Source: CAD feature listing. Evaluate the final solid. Frame: model axes, mm. Round coordinates to 2 decimals unless told otherwise and drop trailing zeros. Write each loop counter-clockwise with the first axis right and the second up, starting at its lowest first coordinate (ties: lowest second). Pieces come first, ordered by that corner, then holes. Notation, with made-up numbers: M 5,54 L 11,54 A18 ccw 11,83 Z; hole C 65,87.5 d2. An arc over 180 degrees is marked long. Answer in a Markdown table with one row per item. Add a question column.
Item 1: Cut plane B-B on z = 32. Return loops of the section in (x, y), and give its area (3 significant figures).
Item 2: Cut plane C-C on x = -46. Return loops of the section in (y, z), and give its area (3 significant figures).
Item 3: Material intervals for probe 1 along Z at (x, y) = (-29.5, -34); probe 2 along Z at (x, y) = (-50.5, -35.5); probe 3 along X at (y, z) = (-30, 29), sorted ascending.
Item 4: Contact query for flat-ended pins moving along their axis: pin 1 (4 mm diameter, centred on y = -12.5, z = 26.5, fed in from +X); pin 2 (3 mm diameter, centred on y = -20.5, z = 32, fed in from +X); pin 3 (10 mm diameter, centred on x = -28.5, y = -29, fed in from +Z). Output: stop coordinate, or through.
Item 5: Cut plane A-A on y = -12. Return loops of the section in (x, z), and give its area (3 significant figures).
from build123d import *

# Parameters (mm, degrees)
F0_W     = 25.4
F0_H     = 63.5
F1_DEPTH = 38.1


# Not quite as in the source:
# - a feature names something its author has since deleted; it is built from what else it names


with BuildPart() as f1:
    # F0 (on Front) → F1 (new body)
    with BuildSketch(Plane.XZ):
        Polygon((-101.6, 63.5), (-101.6, 0), (-29.9632605165, 0), (0, 0), (0, 12.7), align=None)
        with Locations((-114.3, 31.75)):
            Rectangle(F0_W, F0_H)
    extrude(amount=F1_DEPTH)


solid = f1.part
Results below:
| question | item | result |
|---|---|---|
| 1 | outline | M -127,-38.1 L -38.6,-38.1 L -38.6,0 L -127,0 Z |
| 1 | area | 3,370 mm2 |
| 2 | outline | M -38.1,0 L 0,0 L 0,35.7 L -38.1,35.7 Z |
| 2 | area | 1,360 mm2 |
| 3 | probe 1 | 0 to 27.45 |
| 3 | probe 2 | 0 to 37.95 |
| 3 | probe 3 | -127 to -32.6 |
| 4 | pin 1 | x = -23.6 |
| 4 | pin 2 | x = -35.6 |
| 4 | pin 3 | z = 29.45 |
| 5 | outline | M -127,0 L 0,0 L 0,12.7 L -101.6,63.5 L -127,63.5 Z |
| 5 | area | 5,480 mm2 |
